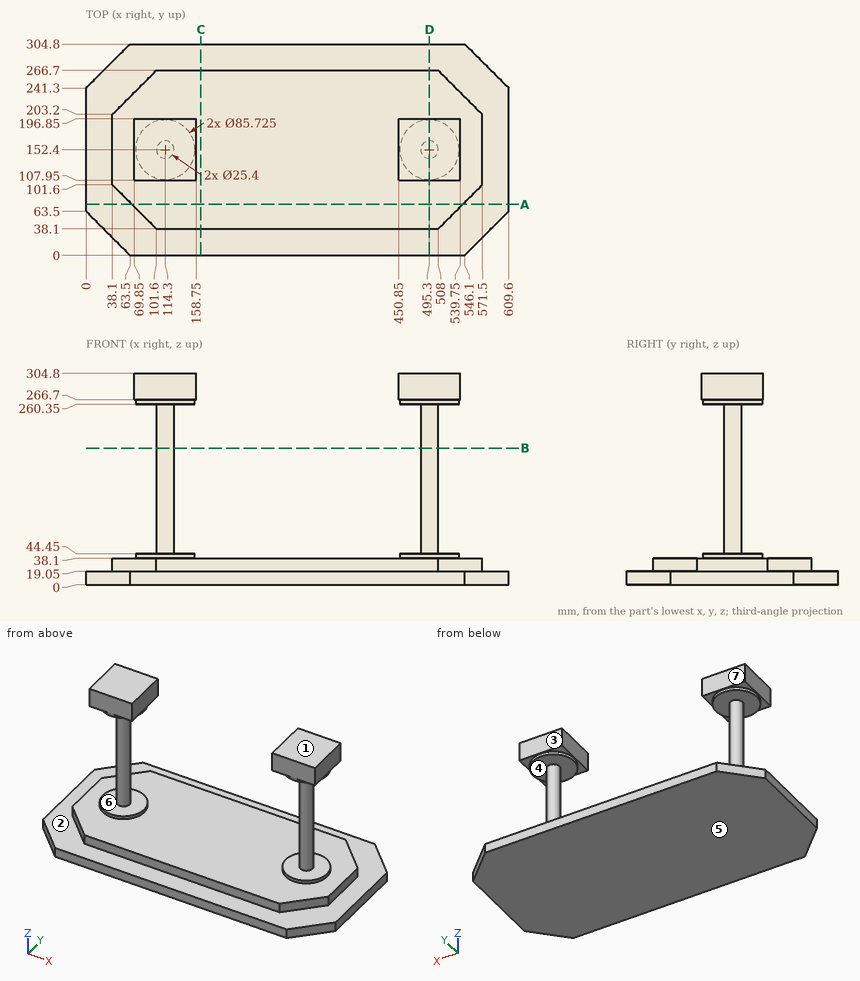
For this review, use the dimensioned drawing (mm, ordinates from the lowest corner) and the shaded views. A direction names the side the tool comes from. Give positions to 0.01 mm unless a question says otherwise; leave off trailing zeros. Loops run counter-clockwise (first coordinate to the right, second up) from the corner with the lowest first, then second, coordinate; pieces in that order, holes last.
Item 1: For line 1 along Z through (x, y) = (196.5, 59); line 2 along X through (y, z) = (152.5, 260); line 3 along Y through (x, z) = (110.5, 288.5), list the stretches that pass through material, from the lowest coordinate up.
Item 2: Insertion check: pin 1 (9.5 mm diameter, centred on y = 144.5, z = 28.5, fed in from -X); pin 2 (4 mm diameter, centred on y = 142, z = 143.5, fed in from -X); pin 3 (1 mm diameter, centred on y = 145.5, z = 56, fed in from +X). Each pin has a flat end and moves straight along its axis. Give the tip position at first contact, or say it passes through.
Item 3: Tool access review of the marked faces 1, 2, 3, 4 and 5: name each direction out of +Z, -Z, +X, -X, +Y, -Y from which nothing blocks a thin tool from reaching the whole face with its end or side.
Item 4: Draft analysis for pull direction X (two halves, no side actions). For the marked faces 6 and 7, state which applies: +X half, -X half, draft (parallel to the pull), parting line (faces both ways), or undercut.
Item 5: Take a section at B-B, the plane z = 197. State the section outline as (x, y) points, and give its area (3 significant figures).
Item 6: Take a section at C-C, the plane x = 165.5. State the section outline as (y, z) points.
Item 7: Take a section at A-A, the plane y = 73.5. State the section outline as (x, z) points.
Item 8: Take a section at D-D, the plane x = 495.3. State the section outline as (y, z) points, and give its area (3 significant figures).
Calculated:
1. line 1: z = 0 to 38.1
1. line 2: x = 101.6 to 127, 482.6 to 508
1. line 3: y = 107.95 to 196.85
2. pin 1: stops at x = 38.1
2. pin 2: stops at x = 104.77
2. pin 3: stops at x = 506.27
3. face 1: +Z, +X, -X, +Y, -Y
3. face 2: +Z
3. face 3: +Z, +X, -X, +Y
3. face 4: none
3. face 5: -Z, +X, -X, +Y, -Y
4. face 6: undercut
4. face 7: draft
5. outline: circle Ø25.4 at (114.3, 152.4); circle Ø25.4 at (495.3, 152.4)
5. area: 1,010 mm2
6. outline: (0, 0) - (304.8, 0) - (304.8, 19.05) - (266.7, 19.05) - (266.7, 38.1) - (38.1, 38.1) - (38.1, 19.05) - (0, 19.05) - close
7. outline: (0, 0) - (609.6, 0) - (609.6, 19.05) - (543.4, 19.05) - (543.4, 38.1) - (66.2, 38.1) - (66.2, 19.05) - (0, 19.05) - close
8. outline: (0, 0) - (304.8, 0) - (304.8, 19.05) - (266.7, 19.05) - (266.7, 38.1) - (195.26, 38.1) - (195.26, 44.45) - (165.1, 44.45) - (165.1, 260.35) - (195.26, 260.35) - (195.26, 266.7) - (196.85, 266.7) - (196.85, 304.8) - (107.95, 304.8) - (107.95, 266.7) - (109.54, 266.7) - (109.54, 260.35) - (139.7, 260.35) - (139.7, 44.45) - (109.54, 44.45) - (109.54, 38.1) - (38.1, 38.1) - (38.1, 19.05) - (0, 19.05) - close
8. area: 20,100 mm2
